Can you work these out from the drawing? Everything is in mm from the part's minimum corner. A direction names the side the tool comes from. Coordinates: 2 decimals unless noted, no trailing zeros. Loops run counter-clockwise (first coordinate to the right, second up) from the corner with the lowest first, then second, coordinate; pieces in that order, holes last. Notation, with made-up numbers: (36, 38.5) -> (49, 38.5) arc R10 ccw to (49, 45.5) -> close; hole circle Ø11 at (41.25, -29). An arc over 180 degrees is marked (long way). Use one line per item in the form item = value. Start each with the question number.
(1) Imagine slicing it at C-C (x = 7.5). List the corners of the cut face in (y, z) for me.
(2) Imagine slicing it at B-B (y = 11). List the corners of the cut face in (x, z) for me.
(3) I need wall thicknesses on line 1 (Z direction, x = 1.25, y = 8.5); line 2 (X direction, y = 12, z = 4.75) (1 decimal); line 3 (Z direction, x = 16, y = 20.5). Which ranges of each line are inside material? Lowest first, please. Write a range as [from, to].
(4) Imagine slicing it at A-A (z = 5.5). List the corners of the cut face in (x, y) for me.
(5) Thinking about a two-plate mould opening in Y: for the marked faces 3, 4 and 5, which applies, released by +Y, released by -Y, zero draft, split by the parting line, or undercut?
(6) I'm going to push flat-ended pins straight in: pin 1 (3 mm diameter, centred on x = 6, y = 11.5, fed in from -Z); pin 2 (1.5 mm diameter, centred on y = 7.5, z = 1.5, fed in from -X); pin 3 (4 mm diameter, centred on x = 7.5, y = 12.5, fed in from -Z); pin 4 (5 mm diameter, centred on x = 5.5, z = 4, fed in from -Y). Where does each tip first touch, or does it pass through?
(7) On a 3-axis mill with a long thin cutter (end or side, diameter ignored), from which of +Z, -Z, +X, -X, +Y, -Y can I reach the whole of each face in a straight line? I mean the marked faces 1 and 2. Say none if no direction works.
(8) Imagine slicing it at D-D (y = 20.75). List the corners of the cut face in (x, z) for me.
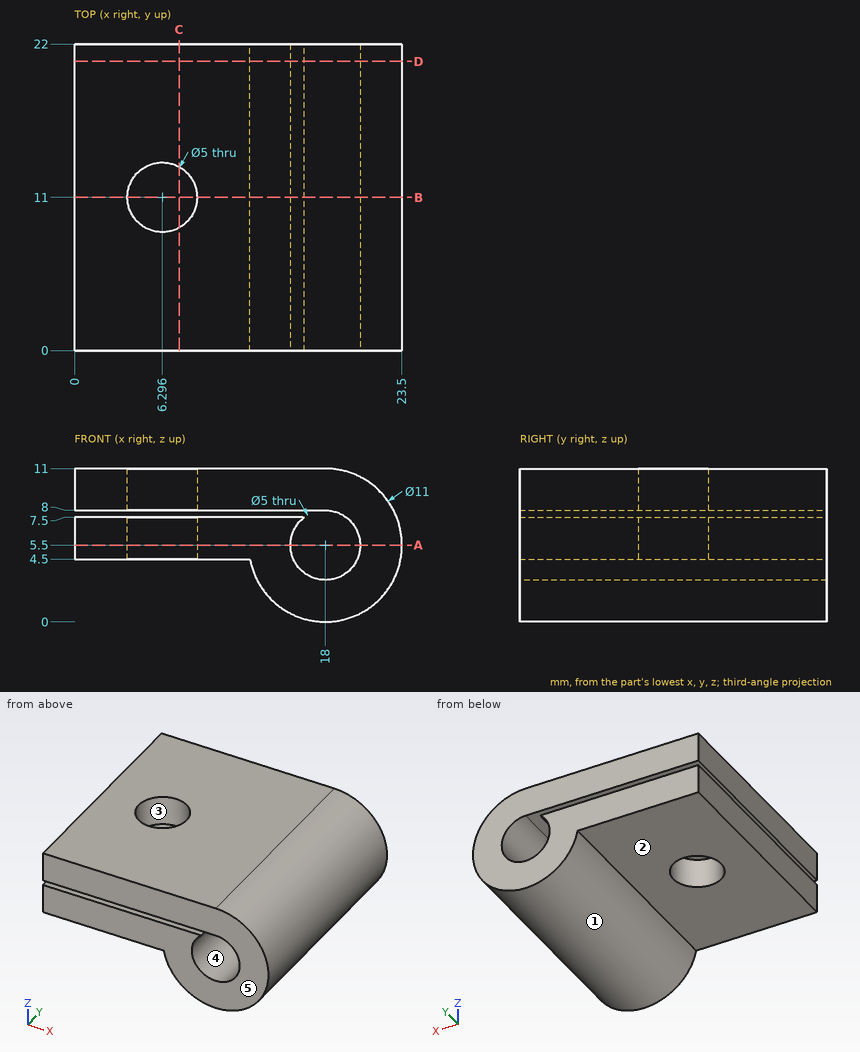
Worked out:
q1.outline = (0, 4.5) -> (8.81, 4.5) -> (8.81, 7.5) -> (0, 7.5) -> close; (0, 8) -> (8.81, 8) -> (8.81, 11) -> (0, 11) -> close; (13.19, 4.5) -> (22, 4.5) -> (22, 7.5) -> (13.19, 7.5) -> close; (13.19, 8) -> (22, 8) -> (22, 11) -> (13.19, 11) -> close
q2.outline = (0, 4.5) -> (3.8, 4.5) -> (3.8, 7.5) -> (0, 7.5) -> close; (0, 8) -> (3.8, 8) -> (3.8, 11) -> (0, 11) -> close; (8.8, 4.5) -> (12.59, 4.5) arc R5.5 ccw (long way) to (18, 11) -> (8.8, 11) -> (8.8, 8) -> (18, 8) arc R2.5 cw (long way) to (16.5, 7.5) -> (8.8, 7.5) -> close
q3.line_1 = [4.5, 7.5], [8, 11]
q3.line_2 = [0, 4], [8.6, 15.6], [20.4, 23.4]
q3.line_3 = [0.38, 4], [7, 7.5], [8, 11]
q4.outline = (0, 0) -> (15.5, 0) -> (15.5, 22) -> (0, 22) -> close; (20.5, 0) -> (23.5, 0) -> (23.5, 22) -> (20.5, 22) -> close; hole circle Ø5 at (6.3, 11)
q5.face_3 = undercut
q5.face_4 = zero draft
q5.face_5 = released by -Y
q6.pin_1 = through
q6.pin_2 = 13.56
q6.pin_3 = 4.5
q6.pin_4 = 0
q7.face_1 = +Y, -Y
q7.face_2 = -Z, -X, +Y, -Y
q8.outline = (0, 4.5) -> (12.59, 4.5) arc R5.5 ccw (long way) to (18, 11) -> (0, 11) -> (0, 8) -> (18, 8) arc R2.5 cw (long way) to (16.5, 7.5) -> (0, 7.5) -> close
